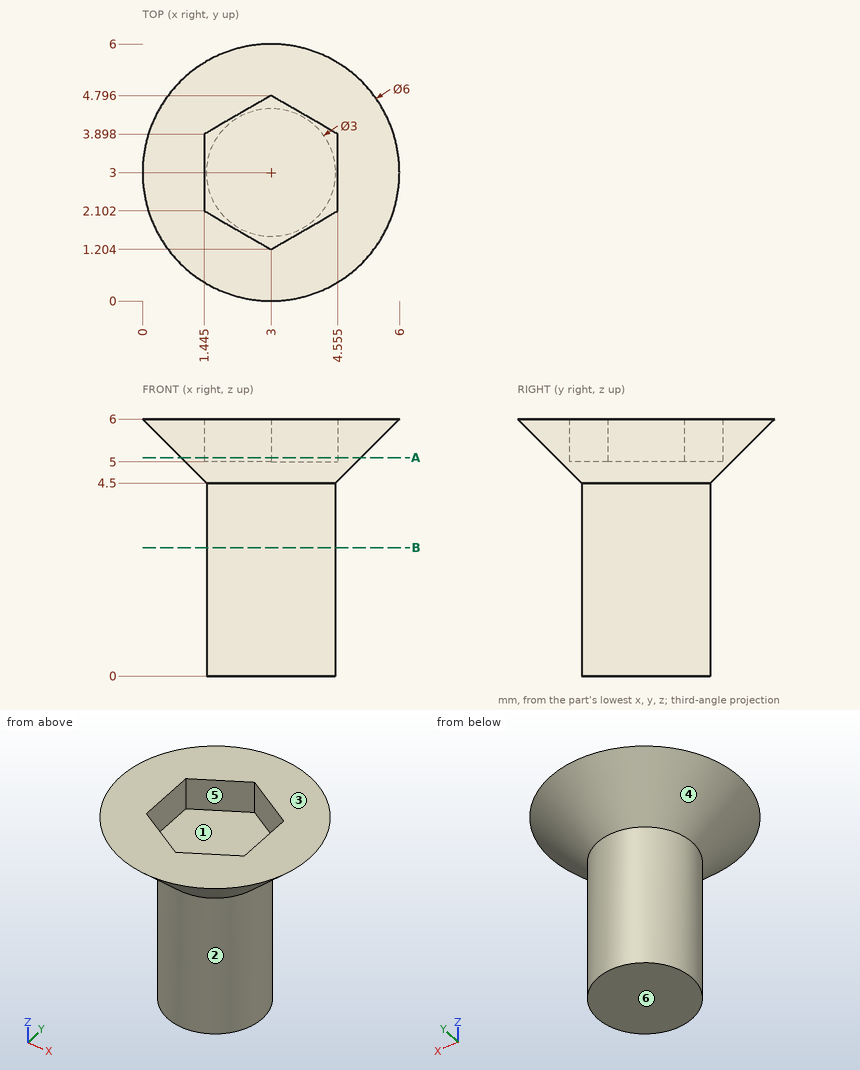
Part print with two shaded views. Sizes in mm from the minimum x, y, z corner. A direction names the side the tool comes from. Coordinates: 2 decimals unless noted, no trailing zeros. Order: outer loops, then holes, each group sorted by start corner. A loop starts at its lowest first (then second) coordinate and runs counter-clockwise, first axis right, second up. Notation, with made-up numbers: (-35, -10) - (-29, -10) arc R25 ccw to (-29, 28) - close; hole circle Ø3 at (-33.75, -2). An arc over 180 degrees is marked (long way). Write item = value, one per line. Start each with the question number.
1) Two-plate mould, pull along X, no slides. Class the marked faces 4, 5 and 6: pulls with the +X half, pulls with the -X half, needs draft (parallel to the pull), parting line crosses it, or undercut.
2) Saw through at B-B on z = 3. Write the cut outline in (x, y).
3) Saw through at A-A on z = 5.1. Write the cut outline in (x, y) (1 decimal).
4) 3-axis set-ups, long thin cutter, end or side, ignore diameter. For the marked faces 1, 2 and 3: which of +Z, -Z, +X, -X, +Y, -Y reach the whole face in a straight line?
5) Wall check: line 1 along Z through (x, y) = (2.8, 4.25); line 2 along Y through (x, z) = (2.5, 5.15) (1 decimal); line 3 along Y through (x, z) = (3, 1.2). Give the ranges that are in metal, low to high. Write a range as from..to.
6) Flat gauge pins, fed straight in: pin 1 Ø2.5 at (x, y) = (4, 3.5) entering from +Z; pin 2 Ø2 at (y, z) = (3, 3) entering from +X; pin 3 Ø2 at (x, z) = (4, 2) entering from -Y. Where does each tip first touch, or does it go through?
From the geometry:
q1.face_4 = parting line crosses it
q1.face_5 = undercut
q1.face_6 = needs draft
q2.outline = circle Ø3 at (3, 3)
q3.outline = circle Ø4.2 at (3, 3); hole (1.4, 2.1) - (3, 1.2) - (4.6, 2.1) - (4.6, 3.9) - (3, 4.8) - (1.4, 3.9) - close
q4.face_1 = +Z
q4.face_2 = -Z
q4.face_3 = +Z, +X, -X, +Y, -Y
q5.line_1 = 0..5
q5.line_2 = 0.9..1.5, 4.5..5.1
q5.line_3 = 1.5..4.5
q6.pin_1 = 6
q6.pin_2 = 4.5
q6.pin_3 = 1.5
